Could you check a few things on this drawing? It's one solid part, dimensions in mm from its lowest x, y, z. A direction names the side the tool comes from. Coordinates: 2 decimals unless noted, no trailing zeros. Order: outer loops, then holes, each group sorted by start corner. A loop starts at its lowest first (then second) coordinate and runs counter-clockwise, first axis right, second up. Notation, with made-up numbers: (87.25, 15) -> (120.25, 15) arc R26 ccw to (120.25, 35) -> close; hole circle Ø8 at (-4, -1). An arc over 180 degrees is marked (long way). Use a Markdown table: item, result. Add a question column.
1. Suppose I cut it at B-B, the plane z = 14.5. List the corners of the cut face in (x, y) for me, then the cut area to 3 significant figures.
2. For pin 1 Ø4 at (x, z) = (2, 18.5) entering from -Y; pin 2 Ø2.5 at (y, z) = (1, 4.5) entering from -X; pin 3 Ø0.9 at (y, z) = (2, 4) entering from +X, each with a flat end and sliding along its axis, tell me the tip position at first contact or that it passes through.
3. For the marked faces 1 and 2, which set-ups out of +Z, -Z, +X, -X, +Y, -Y let a thin tool reach every point of the face, with its end or its side?
4. If I drill on line 1 along Y through (x, z) = (8, 17); line 2 along Z through (x, y) = (8.25, 2.8); line 3 along X through (y, z) = (2.25, 2.5), over which ranges is the centre line in solid material (lowest first)? Write a range as from..to.
5. Suppose I cut it at A-A, the plane y = 2.7. List the corners of the cut face in (x, z) for me.
6. We'd pull the mould along Z, two halves only. Please class the marked faces 3, 4 and 5: pulls with the +Z half, pulls with the -Z half, needs draft (parallel to the pull), parting line crosses it, or undercut.
7. Suppose I cut it at C-C, the plane y = 4.9. List the corners of the cut face in (x, z) for me, then the cut area to 3 significant figures.
8. Suppose I cut it at D-D, the plane x = 3.5. List the corners of the cut face in (y, z) for me.
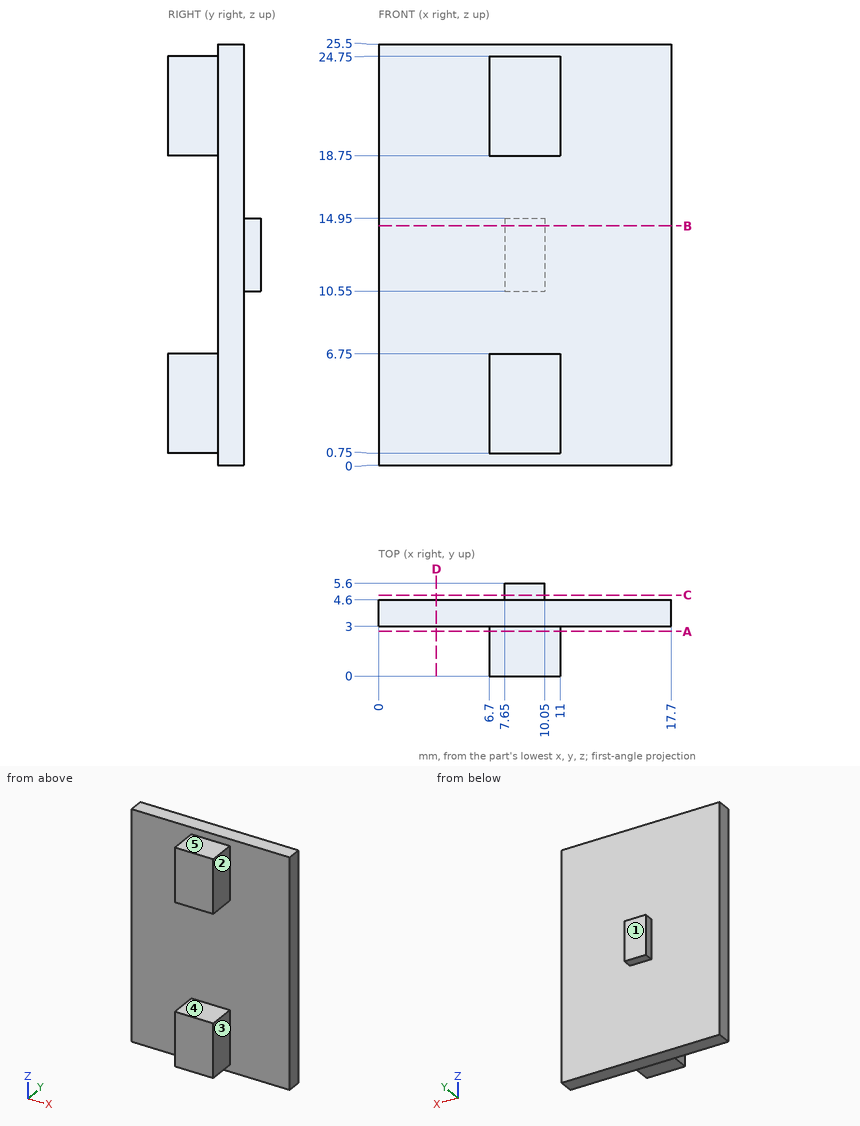
Worked out:
| question | item | result |
|---|---|---|
| 1 | outline | (0, 3) -> (17.7, 3) -> (17.7, 4.6) -> (10.05, 4.6) -> (10.05, 5.6) -> (7.65, 5.6) -> (7.65, 4.6) -> (0, 4.6) -> close |
| 1 | area | 30.7 mm² |
| 2 | pin 1 | stops at y = 3 |
| 2 | pin 2 | stops at x = 6.7 |
| 2 | pin 3 | stops at x = 11 |
| 3 | face 1 | +Z, -Z, +X, -X, +Y |
| 3 | face 2 | +Z, -Z, +X, -Y |
| 4 | line 1 | y = 3..4.6 |
| 4 | line 2 | z = 0.75..6.75, 18.75..24.75 |
| 4 | line 3 | x = 6.7..11 |
| 5 | outline | (6.7, 0.75) -> (11, 0.75) -> (11, 6.75) -> (6.7, 6.75) -> close; (6.7, 18.75) -> (11, 18.75) -> (11, 24.75) -> (6.7, 24.75) -> close |
| 6 | face 3 | needs draft |
| 6 | face 4 | undercut |
| 6 | face 5 | pulls with the +Z half |
| 7 | outline | (7.65, 10.55) -> (10.05, 10.55) -> (10.05, 14.95) -> (7.65, 14.95) -> close |
| 7 | area | 10.6 mm² |
| 8 | outline | (3, 0) -> (4.6, 0) -> (4.6, 25.5) -> (3, 25.5) -> close |
